from build123d import *

# Parameters (mm, degrees)
SKETCH1_W           = 15
SKETCH1_H           = 6
BOSS_EXTRUDE1_DEPTH = 3
CUT_EXTRUDE1_REACH  = 18.432
SKETCH2_R           = 1
SKETCH3_W           = 3
SKETCH3_H           = 6
BOSS_EXTRUDE2_DEPTH = 31
SKETCH4_W           = 6
SKETCH4_H           = 34
BOSS_EXTRUDE3_DEPTH = 1
SKETCH5_W           = 8
SKETCH5_H           = 6
BOSS_EXTRUDE4_DEPTH = 1
SKETCH6_W           = 2
SKETCH6_H           = 15
BOSS_EXTRUDE5_DEPTH = 6


with BuildPart() as part:
    # Sketch1 → Boss-Extrude1 (new body)
    with BuildSketch(Plane(origin=(0, 0, 0), x_dir=(1, 0, 0), z_dir=(0, 1, 0))):
        with Locations((7.5, -3)):
            Rectangle(SKETCH1_W, SKETCH1_H)
    extrude(amount=BOSS_EXTRUDE1_DEPTH)

    # Sketch2 → Cut-Extrude1 (cut, up to next)
    with BuildSketch(Plane(origin=(0, 3, 0), x_dir=(1, 0, 0), z_dir=(0, 1, 0)), mode=Mode.PRIVATE) as cut_extrude1_sk1:
        with Locations(Location((3.25, -2.733160164, 0), (0, 0, 270))):
            Circle(SKETCH2_R)
    cut_extrude1_tool1 = extrude(cut_extrude1_sk1.sketch, amount=-CUT_EXTRUDE1_REACH, mode=Mode.PRIVATE) & part.part
    add(cut_extrude1_tool1.solids().sort_by_distance((3.25, 3, 2.73316))[0], mode=Mode.SUBTRACT)

    # Sketch3 → Boss-Extrude2 (add)
    with BuildSketch(Plane.XZ):
        with Locations((13.5, 3)):
            Rectangle(SKETCH3_W, SKETCH3_H)
    extrude(amount=BOSS_EXTRUDE2_DEPTH)

    # Sketch4 → Boss-Extrude3 (add)
    with BuildSketch(Plane(origin=(15, 0, 0), x_dir=(0, 0, -1), z_dir=(1, 0, 0))):
        with Locations((-3, -14)):
            Rectangle(SKETCH4_W, SKETCH4_H)
    extrude(amount=BOSS_EXTRUDE3_DEPTH)

    # Sketch5 → Boss-Extrude4 (add)
    with BuildSketch(Plane(origin=(0, 3, 0), x_dir=(1, 0, 0), z_dir=(0, 1, 0))):
        with Locations((12, -3)):
            Rectangle(SKETCH5_W, SKETCH5_H)
    extrude(amount=BOSS_EXTRUDE4_DEPTH)

    # Sketch6 → Boss-Extrude5 (add)
    with BuildSketch(Plane.XY):
        with Locations((11, -7.5)):
            Rectangle(SKETCH6_W, SKETCH6_H)
    extrude(amount=BOSS_EXTRUDE5_DEPTH)


solid = part.part
The model under review builds one solid part; all positions refer to its coordinate system, in mm. A direction names the side the tool comes from. Round coordinates to 2 decimals unless told otherwise and drop trailing zeros. Loops run counter-clockwise (first coordinate to the right, second up) from the corner with the lowest first, then second, coordinate; pieces in that order, holes last. Notation, with made-up numbers: (-36.75, 37.5) -> (8.25, 37.5) arc R12 ccw to (8.25, 57.5) -> close; hole circle Ø9 at (-26.75, 26). An arc over 180 degrees is marked (long way). Return JSON: item names as keys, results as strings.
(1) Add section A-A on x = 3.25. Write out the cut boundary in (y, z).
Solved:
{"outline": "(0, 0) -> (3, 0) -> (3, 1.73) -> (0, 1.73) -> close; (0, 3.73) -> (3, 3.73) -> (3, 6) -> (0, 6) -> close"}
(2) For line 1 (X direction, y = -28, z = 5.15); line 2 (X direction, y = -8, z = 1.2); line 3 (Y direction, x = 2.25, z = 4.65), list the stretches that pass through material, from the lowest coordinate up.
Solved:
{"line 1": "12 to 16", "line 2": "10 to 16", "line 3": "0 to 3"}
(3) Add section C-C on z = 4.4. Write out the cut boundary in (x, y).
Solved:
{"outline": "(0, 0) -> (10, 0) -> (10, -15) -> (12, -15) -> (12, -31) -> (16, -31) -> (16, 4) -> (8, 4) -> (8, 3) -> (0, 3) -> close"}
(4) Add section D-D on y = -1. Write out the cut boundary in (x, z), plus the area to 3 significant figures.
Solved:
{"outline": "(10, 0) -> (16, 0) -> (16, 6) -> (10, 6) -> close", "area": "36.0 mm2"}
(5) For pin 1 (0.5 mm diameter, centred on y = 3.5, z = 2.5, fed in from -X); pin 2 (1.5 mm diameter, centred on x = 7.5, z = 3.5, fed in from -Y); pin 3 (0.6 mm diameter, centred on x = 10.5, z = 4, fed in from -Y); pin 4 (2 mm diameter, centred on x = 7.5, y = 0.5, fed in from -Z), all flat-tipped, find the tip position at first contact; note any pin that passes through.
Solved:
{"pin 1": "x = 8", "pin 2": "y = 0", "pin 3": "y = -15", "pin 4": "z = 0"}
(6) Add section B-B on z = 2.55. Write out the cut boundary in (x, y), plus the area to 3 significant figures.
Solved:
{"outline": "(0, 0) -> (2.27, 0) -> (2.27, 3) -> (0, 3) -> close; (4.23, 0) -> (10, 0) -> (10, -15) -> (12, -15) -> (12, -31) -> (16, -31) -> (16, 4) -> (8, 4) -> (8, 3) -> (4.23, 3) -> close", "area": "204 mm2"}
(7) For faces 1 (the flat face through (8, 3.5, 3)), 2 (the flat face through (14, -31, 3)), 3 (the flat face through (5, 0, 3)), list the 3-axis set-ups (+Z, -Z, +X, -X, +Y, -Y) from which the entire face can be reached by the end or side of a thin tool; tool diameter is ignored.
Solved:
{"face 1": "+Z, -Z, -X, +Y", "face 2": "+Z, -Z, +X, -X, -Y", "face 3": "+Z, -Z, -X, -Y"}
